```python
from build123d import *

# Parameters (mm, degrees)
SALIENTE_EXTRUIR1_DEPTH                              = 25
REDONDEO1_R                                          = 10
REDONDEO2_R                                          = 3
CROQUIS2_R                                           = 1.5
CORTAR_EXTRUIR1_DEPTH                                = 9
REFRENTADO_PARA_TORNILLO_TAP_N_CON_CABEZ_D           = 3.4
REFRENTADO_PARA_TORNILLO_TAP_N_CON_CABEZ_CSINK_D     = 6.72
REFRENTADO_PARA_TORNILLO_TAP_N_CON_CABEZ_CSINK_ANGLE = 90
CROQUIS5_W                                           = 40
CROQUIS5_H                                           = 2
CORTAR_EXTRUIR2_DEPTH                                = 25


with BuildPart() as part:
    # Croquis1 → Saliente-Extruir1 (new body)
    with BuildSketch(Plane.XY):
        Polygon((-96.521895292, -23.642699491), (-136.521895292, -23.642699491), (-136.521895292, -14.642699491), (-106.521895292, -14.642699491), (-106.521895292, 16.357300509), (-1.521895292, 16.357300509), (-1.521895292, -14.642699491), (28.478104708, -14.642699491), (28.478104708, -23.642699491), (-11.521895292, -23.642699491), (-11.521895292, 1.357300509), (-96.521895292, 1.357300509), align=None)
    extrude(amount=SALIENTE_EXTRUIR1_DEPTH)

    # Redondeo1
    redondeo1_edges = [part.edges().sort_by_distance(p)[0] for p in [
        (-54.021895292, 1.357300509, 0),
        (-54.021895292, 1.357300509, 25),
    ]]
    fillet(redondeo1_edges, radius=REDONDEO1_R)

    # Redondeo2
    redondeo2_edges = [part.edges().sort_by_distance(p)[0] for p in [
        (-54.021895292, 16.357300509, 0),
    ]]
    fillet(redondeo2_edges, radius=REDONDEO2_R)

    # Croquis2 → Cortar-Extruir1 (cut)
    with BuildSketch(Plane(origin=(0, -14.642699491, 0), x_dir=(1, 0, 0), z_dir=(0, 1, 0))):
        with Locations((-113.521895292, -12.5)):
            Circle(CROQUIS2_R)
        with Locations((-128.521895292, -12.5)):
            Circle(CROQUIS2_R)
        with Locations((20.478104708, -12.5)):
            Circle(CROQUIS2_R)
        with Locations((5.478104708, -12.5)):
            Circle(CROQUIS2_R)
    extrude(amount=-CORTAR_EXTRUIR1_DEPTH, mode=Mode.SUBTRACT)

    # Refrentado para tornillo tapón con cabeza plana de clavija de M31 (through all)
    with Locations(Plane(origin=(0, -14.642699491, 0), x_dir=(1, 0, 0), z_dir=(0, 1, 0))):
        with Locations((-128.521895292, -12.5), (-113.521895292, -12.5), (20.478104708, -12.5), (5.478104708, -12.5)):
            CounterSinkHole(REFRENTADO_PARA_TORNILLO_TAP_N_CON_CABEZ_D / 2, REFRENTADO_PARA_TORNILLO_TAP_N_CON_CABEZ_CSINK_D / 2, counter_sink_angle=REFRENTADO_PARA_TORNILLO_TAP_N_CON_CABEZ_CSINK_ANGLE)

    # Croquis5 → Cortar-Extruir2 (cut)
    with BuildSketch(Plane.XY.offset(25)):
        with Locations((-116.521895292, -22.642699491)):
            Rectangle(CROQUIS5_W, CROQUIS5_H)
        with Locations((8.478104708, -22.642699491)):
            Rectangle(CROQUIS5_W, CROQUIS5_H)
    extrude(amount=-CORTAR_EXTRUIR2_DEPTH, mode=Mode.SUBTRACT)


solid = part.part
```
Verification items for the finished model (mm, model axes). A direction names the side the tool comes from. Round coordinates to 2 decimals unless told otherwise and drop trailing zeros. Write each loop counter-clockwise with the first axis right and the second up, starting at its lowest first coordinate (ties: lowest second). Pieces come first, ordered by that corner, then holes. Notation, with made-up numbers: (34.5, 79.25) -> (50.5, 79.25) arc R12 cw to (50.5, 85.25) -> close; hole circle Ø7 at (-0.75, 81.5). An arc over 180 degrees is marked (long way). Write each question's results on one line, items separated by ' | '. Start each with the question number.
1. Cross-section at C-C (z = 12.5). Count the separate pieces of the cut face and the enclosed holes in it, then the cut area to 3 significant figures.
2. Cross-section at B-B (x = -70). Enter the section's corners in (y, z), then the cut area to 3 significant figures.
3. Cross-section at D-D (y = 3.5). Enter the section's corners in (x, z).
4. Cross-section at A-A (y = -4). Enter the section's corners in (x, z), then the cut area to 3 significant figures.
5. Material ranges on probe 1 along X at (y, z) = (-20.05, 12.5); probe 2 along X at (y, z) = (-15, 12); probe 3 along X at (y, z) = (-17.5, 8.5), recorded low to high. Write a range as from..to.
6. Draft check along Z on faces 1 (the cylindrical face through (22.176, -19.01, 12.425)), 2 (the cylindrical face through (-115.143, -19.01, 11.989)), 3 (the flat face through (-55, 16.357, 14)), 4 (the flat face through (-48, 13, 25)). Enter one of: +Z half, -Z half, draft (parallel to the pull), parting line (faces both ways), or undercut.
7. Depth check by flat-ended pin: P1, Ø5, axis at x = -57, z = 18.5, coming from the -Y side; P2, Ø8, axis at y = -10.5, z = 13.5, coming from the -X side; P3, Ø10, axis at x = -21, y = 0, coming from the -Z side. Enter the tip coordinate at first touch or a pass-through.
8. Set-up check for faces 5 (the flat face through (-1.522, 1, 12)), 6 (the cylindrical face through (-54.617, 4.209, 21.993)), 7 (the cylindrical face through (-54.617, 4.209, 3.007)): record each of +Z, -Z, +X, -X, +Y, -Y from which the full face is reachable in a straight line by a thin tool's end or side.
Solutions:
1) separate pieces: 5 | enclosed holes: 0 | area: 2,350 mm2
2) outline: (1.36, 10) arc R10 ccw to (11.36, 0) -> (13.36, 0) arc R3 ccw to (16.36, 3) -> (16.36, 25) -> (11.36, 25) arc R10 ccw to (1.36, 15) -> close | area: 330 mm2
3) outline: (-106.52, 0) -> (-96.52, 0) -> (-96.52, 3.81) -> (-11.52, 3.81) -> (-11.52, 0) -> (-1.52, 0) -> (-1.52, 25) -> (-11.52, 25) -> (-11.52, 21.19) -> (-96.52, 21.19) -> (-96.52, 25) -> (-106.52, 25) -> close
4) outline: (-106.52, 0) -> (-96.52, 0) -> (-96.52, 25) -> (-106.52, 25) -> close; (-11.52, 0) -> (-1.52, 0) -> (-1.52, 25) -> (-11.52, 25) -> close | area: 500 mm2
5) probe 1: x = -136.52..-130.22, -126.82..-115.22, -111.82..-96.52, -11.52..3.78, 7.18..18.78, 22.18..28.48 | probe 2: x = -136.52..-131.48, -125.56..-116.48, -110.56..-96.52, -11.52..2.52, 8.44..17.52, 23.44..28.48 | probe 3: x = -136.52..-96.52, -11.52..28.48
6) face 1: undercut | face 2: undercut | face 3: draft | face 4: +Z half
7) P1: stops at y = 1.41 | P2: stops at x = -106.52 | P3: stops at z = 2.28
8) face 5: +Z, -Z, +X, +Y | face 6: +Z, -Y | face 7: -Z, -Y
